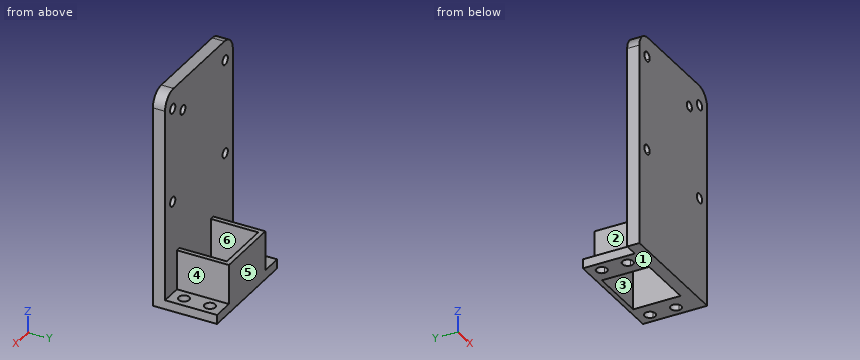
```python
from build123d import *

# Parameters (mm, degrees)
F0_W      = 40
F0_H      = 71
F1_DEPTH  = 4
F3_DEPTH  = 25
F4_W      = 21.5
F4_H      = 16
F5_DEPTH  = 17
F6_W      = 18.5
F6_H      = 15.5
F7_DEPTH  = 25
F8_W      = 17
F8_H      = 3
F9_DEPTH  = 7
F10_W     = 17
F10_H     = 3
F11_DEPTH = 7
F13_DEPTH = 25
F15_DEPTH = 25
F17_DEPTH = 10
F18_DEPTH = 25
F20_R     = 5
F21_DEPTH = 10
F22_R     = 2.0074769643
F23_DEPTH = 4
F25_DEPTH = 25


with BuildPart() as f1:
    # F0 (on Front) → F1 (new body)
    with BuildSketch(Plane.XZ):
        Rectangle(F0_W, F0_H)
    extrude(amount=F1_DEPTH)

    # F2 (on face) → F3 (cut)
    with BuildSketch(Plane.XZ.offset(4)):
        with BuildLine():
            ThreePointArc((17.05, -2), (15.5, -0.45), (13.95, -2))
            ThreePointArc((13.95, -2), (15.5, -3.55), (17.05, -2))
        make_face()
        with BuildLine():
            ThreePointArc((-13.95, -2), (-14.4039844892, -0.9039844892), (-15.5, -0.45))
            Line((-15.5, -0.45), (-15.5, -2))
            Line((-15.5, -2), (-13.95, -2))
        make_face()
        with BuildLine():
            Line((-15.5, -2), (-15.5, -0.45))
            ThreePointArc((-15.5, -0.45), (-16.5960155108, -3.0960155108), (-13.95, -2))
            Line((-13.95, -2), (-15.5, -2))
        make_face()
        with BuildLine():
            ThreePointArc((-15.5, 27.45), (-14.4039844892, 27.9039844892), (-13.95, 29))
            Line((-13.95, 29), (-15.5, 29))
            Line((-15.5, 29), (-15.5, 27.45))
        make_face()
        with BuildLine():
            Line((-15.5, 29), (-13.95, 29))
            ThreePointArc((-13.95, 29), (-14.4039844892, 30.0960155108), (-15.5, 30.55))
            Line((-15.5, 30.55), (-15.5, 29))
        make_face()
        with BuildLine():
            ThreePointArc((17.05, 29), (15.5, 30.55), (13.95, 29))
            ThreePointArc((13.95, 29), (15.5, 27.45), (17.05, 29))
        make_face()
        with BuildLine():
            Line((-15.5, 27.45), (-15.5, 29))
            Line((-15.5, 29), (-15.5, 30.55))
            ThreePointArc((-15.5, 30.55), (-17.05, 29), (-15.5, 27.45))
        make_face()
    extrude(amount=-F3_DEPTH, mode=Mode.SUBTRACT)

    # F4 (on face) → F5 (join)
    with BuildSketch(Plane(origin=(0, 0, 0), x_dir=(-1, 0, 0), z_dir=(0, 1, 0))):
        with Locations((-2.25, -27.5)):
            Rectangle(F4_W, F4_H)
    extrude(amount=F5_DEPTH)

    # F6 (on face) → F7 (cut)
    with BuildSketch(Plane.XY.offset(-19.5)):
        with Locations((2.25, 7.75)):
            Rectangle(F6_W, F6_H)
    extrude(amount=-F7_DEPTH, mode=Mode.SUBTRACT)

    # F8 (on face) → F9 (join)
    with BuildSketch(Plane.YZ.offset(13)):
        with Locations((8.5, -34)):
            Rectangle(F8_W, F8_H)
    extrude(amount=F9_DEPTH)

    # F10 (on face) → F11 (join)
    with BuildSketch(Plane(origin=(-8.5, 0, 0), x_dir=(0, -1, 0), z_dir=(-1, 0, 0))):
        with Locations((-8.5, -34)):
            Rectangle(F10_W, F10_H)
    extrude(amount=F11_DEPTH)

    # F12 (on face) → F13 (cut)
    with BuildSketch(Plane.XY.offset(-32.5)):
        with BuildLine():
            Line((-12, 14.5), (-12, 11))
            ThreePointArc((-12, 11), (-10.7625631329, 11.5125631329), (-10.25, 12.75))
            ThreePointArc((-10.25, 12.75), (-10.7625631329, 13.9874368671), (-12, 14.5))
        make_face()
        with BuildLine():
            ThreePointArc((-12, 14.5), (-13.75, 12.75), (-12, 11))
            Line((-12, 11), (-12, 14.5))
        make_face()
        with BuildLine():
            ThreePointArc((-12, 6), (-13.75, 4.25), (-12, 2.5))
            Line((-12, 2.5), (-12, 6))
        make_face()
        with BuildLine():
            Line((-12, 6), (-12, 2.5))
            ThreePointArc((-12, 2.5), (-10.7625631329, 3.0125631329), (-10.25, 4.25))
            ThreePointArc((-10.25, 4.25), (-10.7625631329, 5.4874368671), (-12, 6))
        make_face()
    extrude(amount=-F13_DEPTH, mode=Mode.SUBTRACT)

    # F14 (on face) → F15 (cut)
    with BuildSketch(Plane.XY.offset(-32.5)):
        with BuildLine():
            ThreePointArc((18.25, 12.75), (17.7374368671, 13.9874368671), (16.5, 14.5))
            Line((16.5, 14.5), (16.5, 11))
            ThreePointArc((16.5, 11), (17.7374368671, 11.5125631329), (18.25, 12.75))
        make_face()
        with BuildLine():
            ThreePointArc((18.25, 4.25), (17.7374368671, 5.4874368671), (16.5, 6))
            Line((16.5, 6), (16.5, 2.5))
            ThreePointArc((16.5, 2.5), (17.7374368671, 3.0125631329), (18.25, 4.25))
        make_face()
        with BuildLine():
            Line((16.5, 2.5), (16.5, 6))
            ThreePointArc((16.5, 6), (14.75, 4.25), (16.5, 2.5))
        make_face()
        with BuildLine():
            Line((16.5, 11), (16.5, 14.5))
            ThreePointArc((16.5, 14.5), (14.75, 12.75), (16.5, 11))
        make_face()
    extrude(amount=-F15_DEPTH, mode=Mode.SUBTRACT)

    # F16 (on face) → F17 (join)
    with BuildSketch(Plane.XZ.offset(4)):
        Polygon((-20, -25.5), (-20, -35.5), (-15.5, -35.5), (-11, -35.5), (-11, -25.5), align=None)
        with BuildLine():
            ThreePointArc((-13.75, -30.5), (-14.2625631329, -31.7374368671), (-15.5, -32.25))
            ThreePointArc((-15.5, -32.25), (-16.7374368671, -29.2625631329), (-13.75, -30.5))
        make_face(mode=Mode.SUBTRACT)
    extrude(amount=F17_DEPTH)

    # F18 (cut): a face of the model
    f18_faces = [f1.faces().sort_by_distance(p)[0] for p in [
        (-15.5, -4, -30.5),
    ]]
    extrude(f18_faces, amount=-F18_DEPTH, mode=Mode.SUBTRACT)

    # F20
    f20_edges = [f1.edges().sort_by_distance(p)[0] for p in [
        (-20, -2, 35.5),
        (20, -2, 35.5),
    ]]
    fillet(f20_edges, radius=F20_R)

    # F21 (cut): a face of the model
    f21_faces = [f1.faces().sort_by_distance(p)[0] for p in [
        (-19.8654637595, -14, -30.5),
    ]]
    extrude(f21_faces, amount=-F21_DEPTH, mode=Mode.SUBTRACT)

    # F22 (on face) → F23 (join)
    with BuildSketch(Plane.XZ.offset(4)):
        with Locations((-15.5, -30.5)):
            Circle(F22_R)
    extrude(amount=-F23_DEPTH)

    # F24 (on face) → F25 (cut)
    with BuildSketch(Plane.XZ.offset(4)):
        with BuildLine():
            ThreePointArc((9.5, 24), (10.5606601718, 24.4393398282), (11, 25.5))
            ThreePointArc((11, 25.5), (8.4393398282, 26.5606601718), (9.5, 24))
        make_face()
    extrude(amount=-F25_DEPTH, mode=Mode.SUBTRACT)


solid = f1.part
```
The model under review builds one solid part; all positions refer to its coordinate system, in mm. Face numbers are marked on the shaded views. A direction names the side the tool comes from. Round coordinates to 2 decimals unless told otherwise and drop trailing zeros. Loops run counter-clockwise (first coordinate to the right, second up) from the corner with the lowest first, then second, coordinate; pieces in that order, holes last.
Item 1: Clearance check with flat-ended pins moving along their axes: pin 1 Ø4 at (x, z) = (15.5, -2) entering from +Y; pin 2 Ø6.5 at (y, z) = (5, -26.5) entering from -X; pin 3 Ø7.5 at (x, y) = (17.5, 4.5) entering from +Z. State where each tip first meets the part, or that it passes through.
Determined:
pin 1: stops at y = 0
pin 2: stops at x = -8.5
pin 3: stops at z = -32.5
Item 2: Take a section at C-C (z = 17). Write out the cut boundary in (x, y).
Determined:
outline: (-20, -4) - (20, -4) - (20, 0) - (-20, 0) - close
Item 3: Mouldability with a two-part tool opening along X and no side actions: class the marked faces 4, 5 and 6 as released by +X, released by -X, zero draft, split by the parting line, or undercut.
Determined:
face 4: released by +X
face 5: zero draft
face 6: undercut
Item 4: Take a section at B-B (y = 3.5). Write out the cut boundary in (x, z).
Determined:
outline: (-15.5, -35.5) - (-13.58, -35.5) - (-13.58, -32.5) - (-15.5, -32.5) - close; (-10.42, -35.5) - (-7, -35.5) - (-7, -19.5) - (-8.5, -19.5) - (-8.5, -32.5) - (-10.42, -32.5) - close; (11.5, -35.5) - (14.92, -35.5) - (14.92, -32.5) - (13, -32.5) - (13, -19.5) - (11.5, -19.5) - close; (18.08, -35.5) - (20, -35.5) - (20, -32.5) - (18.08, -32.5) - close
Item 5: For line 1 (X direction, y = -0.95, z = -2); line 2 (Y direction, x = -2.5, z = -28.5); line 3 (X direction, y = 8, z = -28.5), list the stretches that pass through material, from the lowest coordinate up.
Determined:
line 1: x = -20 to -17.05, -13.95 to 13.95, 17.05 to 20
line 2: y = -4 to 0, 15.5 to 17
line 3: x = -8.5 to -7, 11.5 to 13
Item 6: Take a section at A-A (x = 1). Write out the cut boundary in (y, z).
Determined:
outline: (-4, -35.5) - (0, -35.5) - (0, 35.5) - (-4, 35.5) - close; (15.5, -35.5) - (17, -35.5) - (17, -19.5) - (15.5, -19.5) - close
Item 7: For the marked faces 1, 2 and 3, list the 3-axis set-ups (+Z, -Z, +X, -X, +Y, -Y) from which the entire face can be reached by the end or side of a thin tool; tool diameter is ignored.
Determined:
face 1: -Z, +X, -X, +Y, -Y
face 2: +Z, -X, +Y
face 3: +Z, -Z
